Study the drawing (mm; zero at the part's minimum x, y, z) and answer. Give positions to 0.01 mm unless a question says otherwise; leave off trailing zeros. Order: outer loops, then holes, each group sorted by start corner. A loop starts at its lowest first (then second) coordinate and runs counter-clockwise, first axis right, second up. Notation, with made-up numbers: (-17.75, -3) - (36.25, -3) arc R11 cw to (36.25, 14) - close; hole circle Ø3 at (-16.75, -30.5). An arc over 180 degrees is marked (long way). Use CSV: the item, a comma, the result in double quotes.
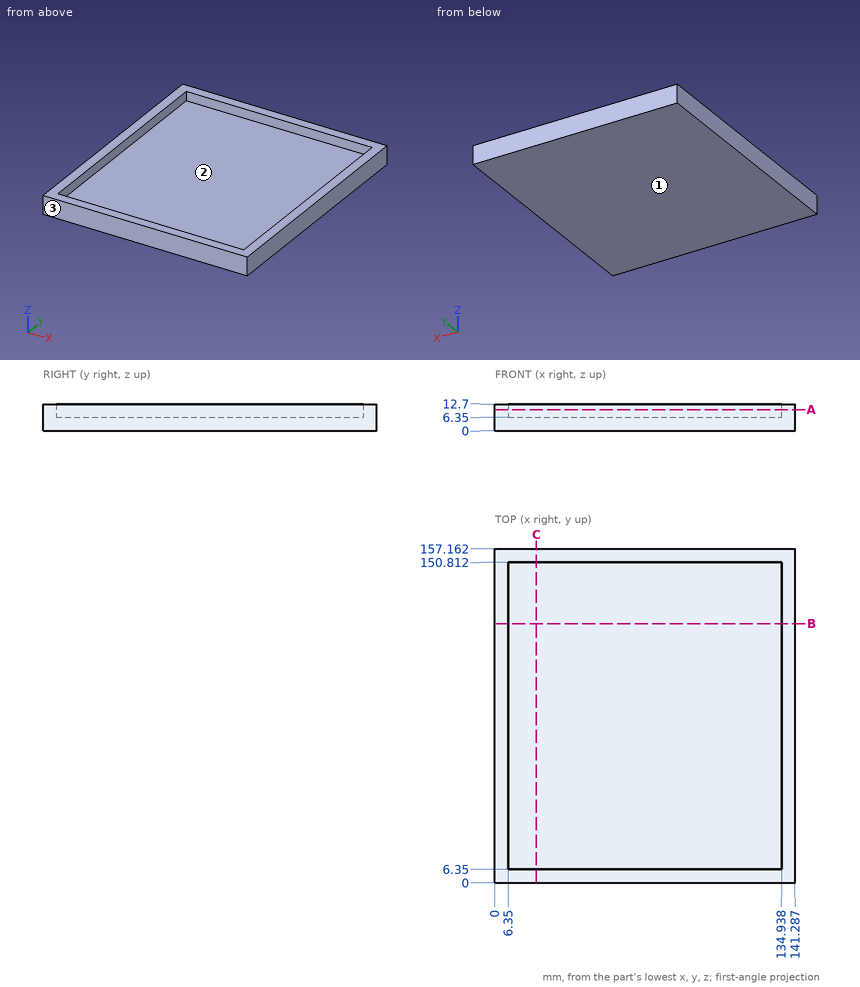
Item 1: The part is cut by section C-C (x = 19.5). Give the vertices of the cut face in (y, z).
Taken from the geometry:
outline,"(0, 0) - (157.16, 0) - (157.16, 12.7) - (150.81, 12.7) - (150.81, 6.35) - (6.35, 6.35) - (6.35, 12.7) - (0, 12.7) - close"
Item 2: The part is cut by section B-B (y = 122). Give the vertices of the cut face in (x, z).
Taken from the geometry:
outline,"(0, 0) - (141.29, 0) - (141.29, 12.7) - (134.94, 12.7) - (134.94, 6.35) - (6.35, 6.35) - (6.35, 12.7) - (0, 12.7) - close"
Item 3: This flat-tipped pin is pushed along its axis until it touches: pin 1 (12 mm diameter, centred on x = 38.5, y = 16.5, fed in from +Z). Where does it stop, or does it pass through?
Taken from the geometry:
pin 1,"z = 6.35"
Item 4: The mould has two halves that part along Y. Classify the marked faces 1, 2 and 3: +Y half, -Y half, draft (parallel to the pull), parting line (faces both ways), or undercut.
Taken from the geometry:
face 1,"draft"
face 2,"undercut"
face 3,"-Y half"
Item 5: Find the intervals of material crossed by line 1 along Y through (x, z) = (27.5, 11.75); line 2 along X through (y, z) = (117.5, 11.5); line 3 along Z through (x, y) = (18.5, 99.5), in increasing order.
Taken from the geometry:
line 1,"0 to 6.35, 150.81 to 157.16"
line 2,"0 to 6.35, 134.94 to 141.29"
line 3,"0 to 6.35"
Item 6: The part is cut by section A-A (z = 10). Give the vertices of the cut face in (x, y), and give its area (3 significant figures).
Taken from the geometry:
outline,"(0, 0) - (141.29, 0) - (141.29, 157.16) - (0, 157.16) - close; hole (6.35, 6.35) - (134.94, 6.35) - (134.94, 150.81) - (6.35, 150.81) - close"
area,"3,630 mm^2"
